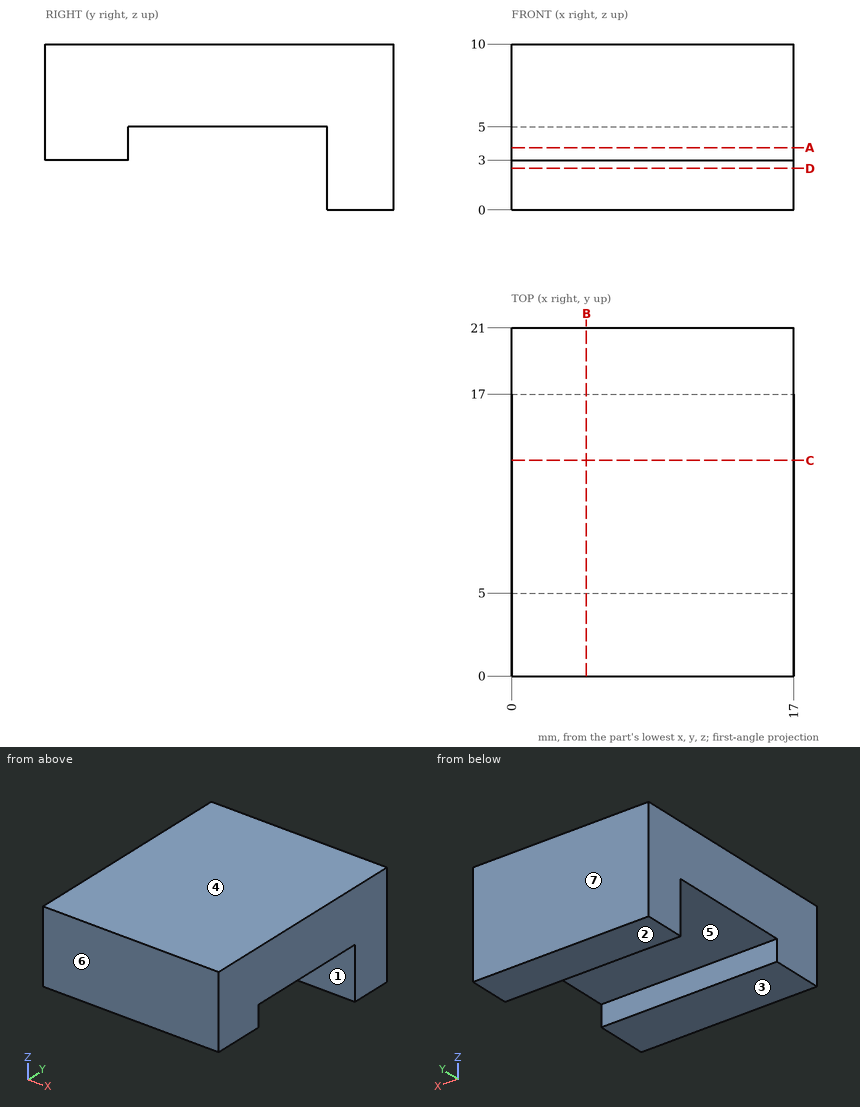
The drawing under review shows one solid part. Ordinate dimensions are in mm from its lowest x, y, z. A direction names the side the tool comes from. Give positions to 0.01 mm unless a question says otherwise; leave off trailing zeros. Write each loop counter-clockwise with the first axis right and the second up, starting at its lowest first coordinate (ties: lowest second). Pieces come first, ordered by that corner, then holes. Notation, with made-up numbers: (1, 7) -> (49, 7) arc R22 ccw to (49, 43) -> close; hole circle Ø8 at (-1, -6.75). An arc over 180 degrees is marked (long way). Put each result on its own line as item: value.
(1) We need section D-D, the plane z = 2.5. Give the boundary of the cut face in (x, y).
Results are:
outline: (0, 17) -> (17, 17) -> (17, 21) -> (0, 21) -> close
(2) We need section C-C, the plane y = 13. Give the boundary of the cut face in (x, z).
Results are:
outline: (0, 5) -> (17, 5) -> (17, 10) -> (0, 10) -> close
(3) We need section B-B, the plane x = 4.5. Give the boundary of the cut face in (y, z), and give its area (3 significant figures).
Results are:
outline: (0, 3) -> (5, 3) -> (5, 5) -> (17, 5) -> (17, 0) -> (21, 0) -> (21, 10) -> (0, 10) -> close
area: 135 mm²
(4) Tool access review of the marked faces 1, 2 and 3: name each direction out of +Z, -Z, +X, -X, +Y, -Y from which nothing blocks a thin tool from reaching the whole face with its end or side.
Results are:
face 1: -Z, +X, -X
face 2: -Z, +X, -X, +Y, -Y
face 3: -Z, +X, -X, -Y
(5) The part is to be moulded in two halves that separate along Y. For the marked faces 4, 5, 6 and 7, say which applies: pulls with the +Y half, pulls with the -Y half, needs draft (parallel to the pull), parting line crosses it, or undercut.
Results are:
face 4: needs draft
face 5: undercut
face 6: pulls with the -Y half
face 7: pulls with the +Y half
(6) For pin 1 Ø3.5 at (x, y) = (6.5, 11.5) entering from -Z; pin 2 Ø2.5 at (x, y) = (12, 2.5) entering from -Z, all flat-tipped, find the tip position at first contact; note any pin that passes through.
Results are:
pin 1: z = 5
pin 2: z = 3
(7) We need section A-A, the plane z = 3.75. Give the boundary of the cut face in (x, y).
Results are:
outline: (0, 0) -> (17, 0) -> (17, 5) -> (0, 5) -> close; (0, 17) -> (17, 17) -> (17, 21) -> (0, 21) -> close
(8) To check wall thickness, follow probe 1 along Y at (x, z) = (11.75, 3.25); probe 2 along Z at (x, y) = (12.5, 8); probe 3 along Y at (x, z) = (13.5, 1). State the ranges of each line that lie inside material, in increasing order. Write a range as from..to.
Results are:
probe 1: 0..5, 17..21
probe 2: 5..10
probe 3: 17..21
